The listing builds one solid part. Answer for the finished solid, in the listing's coordinates (mm). A direction names the side the tool comes from. Give positions to 0.01 mm unless a question says otherwise; leave off trailing zeros. Write each loop counter-clockwise with the first axis right and the second up, starting at its lowest first coordinate (ties: lowest second). Pieces come first, ordered by that corner, then holes. Notation, with made-up numbers: (14, 12) - (46, 12) arc R6 ccw to (46, 23) - close; hole circle Ø8 at (-5, -34.5). An arc over 180 degrees is marked (long way). Answer as CSV lines item,"result". Start each with the question number.
(1) For faces 4 (the face through (48.025, -1, 19)), 5 (the face through (-39.975, -1, 6)), 6 (the face through (36.025, -1, 6)), 7 (the face through (30, 42, -4)), determine the directions among +Z, -Z, +X, -X, +Y, -Y from which every point of the face is accessible in a straight line to the end or side of a thin tool.
(2) Find section A-A (z = 6.5). Write down the section's boundary in (x, y).
(3) Find section C-C (x = -1). Write down the section's boundary in (y, z), then the cut area to 3 significant figures.
(4) Each of these flat-tipped pins is pushed along its axis until it touches: pin 1 Ø6.5 at (x, y) = (42.03, 29) entering from -Z; pin 2 Ø7 at (y, z) = (8.5, 1.5) entering from +X; pin 3 Ø8 at (x, z) = (1, -0.5) entering from -Y; pin 4 Ø1.5 at (y, z) = (31.5, 10.5) entering from -X. Where does it stop, or does it pass through?
(5) Find section B-B (y = -24). Write down the section's boundary in (x, z).
(6) Find section D-D (y = -2). Write down the section's boundary in (x, z).
(7) For a pull along Y with two mould halves and no side action, classify faces 1 (the face through (42, -1, 17.793)), 2 (the face through (-44.631, 31.108, 19.482)), 3 (the face through (-2, -44, -4)) as pulls with the +Y half, pulls with the -Y half, needs draft (parallel to the pull), parting line crosses it, or undercut.
(8) Straight lines are drawn through the part: probe 1 along X at (y, z) = (-13.5, 5.75); probe 2 along Z at (x, y) = (6, 33.5); probe 3 along Z at (x, y) = (-47.5, -39.5). For each, find the intervals that lie inside material, in ascending order.
from build123d import *

# Parameters (mm, degrees)
F1_DEPTH = 44
F2_R     = 2.5
F3_DEPTH = 3.330463
F4_R     = 30
F5_DEPTH = 3
F6_W     = 6.5
F6_H     = 6.5
F7_DEPTH = 3


with BuildPart() as f1:
    # F0 (on Front) → F1 (new body, symmetric)
    with BuildSketch(Plane.XZ):
        Polygon((33.025175, -2.207002), (-1.974825, -2.207002), (-1.974825, -5.207002), (36.025175, -5.207002), (36.025175, 17.792998), (48.025175, 17.792998), (48.025175, 21.123461), (33.025175, 21.123461), align=None)
        Polygon((-1.974825, -5.207002), (-1.974825, -2.207002), (-36.974825, -2.207002), (-36.974825, 21.123461), (-51.974825, 21.123461), (-51.974825, 17.792998), (-39.974825, 17.792998), (-39.974825, -5.207002), align=None)
    extrude(amount=F1_DEPTH, both=True)

    # F2 (on face) → F3 (cut, through all)
    with BuildSketch(Plane.XY.offset(21.123461)):
        with Locations((42.025175, -29)):
            Circle(F2_R)
        with Locations((42.025175, 29)):
            Circle(F2_R)
        with Locations((-45.974825, 29)):
            Circle(F2_R)
        with Locations((-45.974825, -29)):
            Circle(F2_R)
    extrude(amount=-F3_DEPTH, mode=Mode.SUBTRACT)

    # F4 (on face) → F5 (cut, through all)
    with BuildSketch(Plane.XY.offset(-2.207002)):
        with Locations((1.025122, 0.000286)):
            Circle(F4_R)
    extrude(amount=-F5_DEPTH, mode=Mode.SUBTRACT)

    # F6 (on face) → F7 (cut, through all)
    with BuildSketch(Plane.XY.offset(-2.207002)):
        with Locations((-33.724825, 38.75)):
            Rectangle(F6_W, F6_H)
        with Locations((29.775175, 38.75)):
            Rectangle(F6_W, F6_H)
        with Locations((29.775175, -38.75)):
            Rectangle(F6_W, F6_H)
        with Locations((-33.724825, -38.75)):
            Rectangle(F6_W, F6_H)
    extrude(amount=-F7_DEPTH, mode=Mode.SUBTRACT)


solid = f1.part
Result set:
1,face 4,"+Z, -Z, +X, +Y, -Y"
1,face 5,"-Z, -X, +Y, -Y"
1,face 6,"-Z, +X, +Y, -Y"
1,face 7,"+Z, -Z"
2,outline,"(-39.97, -44) - (-36.97, -44) - (-36.97, 44) - (-39.97, 44) - close; (33.03, -44) - (36.03, -44) - (36.03, 44) - (33.03, 44) - close"
3,outline,"(-44, -5.21) - (-29.93, -5.21) - (-29.93, -2.21) - (-44, -2.21) - close; (29.93, -5.21) - (44, -5.21) - (44, -2.21) - (29.93, -2.21) - close"
3,area,"84.4 mm^2"
4,pin 1,"z = 17.79"
4,pin 2,"x = 36.03"
4,pin 3,"y = -44"
4,pin 4,"x = -39.97"
5,outline,"(-51.97, 17.79) - (-39.97, 17.79) - (-39.97, -5.21) - (-16.97, -5.21) - (-16.97, -2.21) - (-36.97, -2.21) - (-36.97, 21.12) - (-51.97, 21.12) - close; (19.02, -5.21) - (36.03, -5.21) - (36.03, 17.79) - (48.03, 17.79) - (48.03, 21.12) - (33.03, 21.12) - (33.03, -2.21) - (19.02, -2.21) - close"
6,outline,"(-51.97, 17.79) - (-39.97, 17.79) - (-39.97, -5.21) - (-28.91, -5.21) - (-28.91, -2.21) - (-36.97, -2.21) - (-36.97, 21.12) - (-51.97, 21.12) - close; (30.96, -5.21) - (36.03, -5.21) - (36.03, 17.79) - (48.03, 17.79) - (48.03, 21.12) - (33.03, 21.12) - (33.03, -2.21) - (30.96, -2.21) - close"
7,face 1,"needs draft"
7,face 2,"undercut"
7,face 3,"pulls with the -Y half"
8,probe 1,"-39.97 to -36.97, 33.03 to 36.03"
8,probe 2,"-5.21 to -2.21"
8,probe 3,"17.79 to 21.12"
